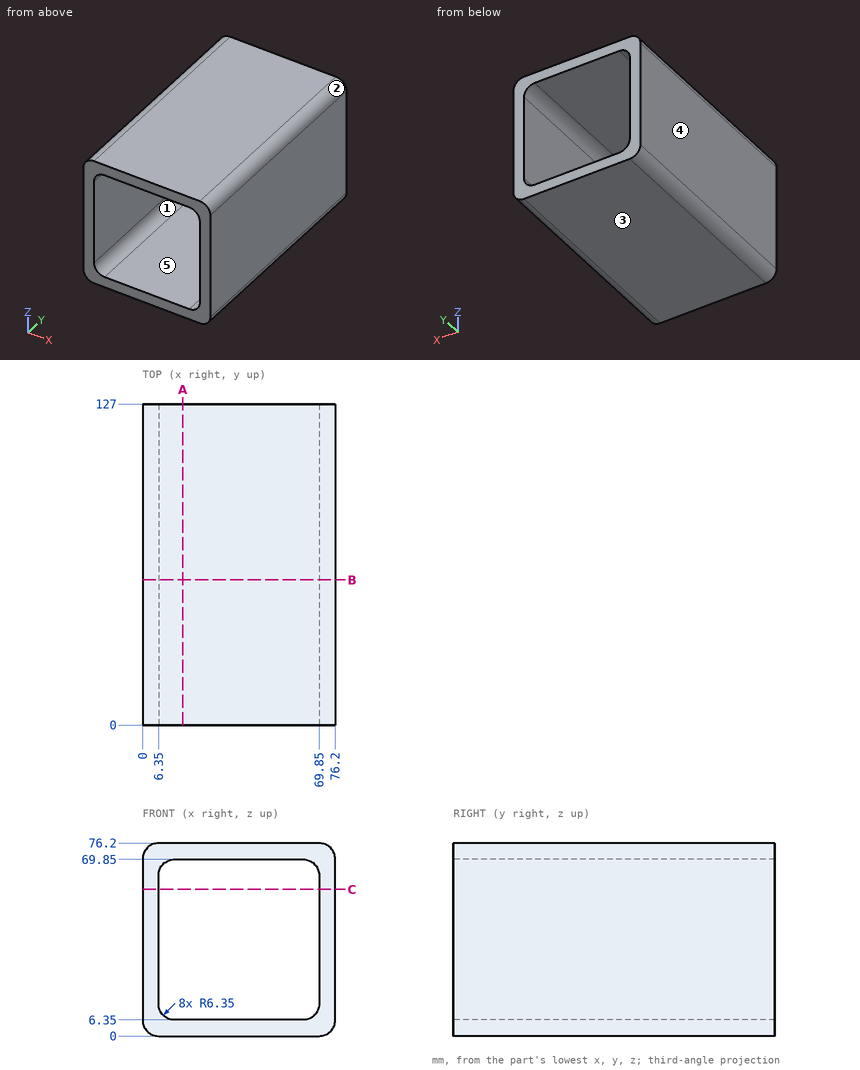
Study the drawing (mm; zero at the part's minimum x, y, z) and answer. A direction names the side the tool comes from. Round coordinates to 2 decimals unless told otherwise and drop trailing zeros. Write each loop counter-clockwise with the first axis right and the second up, starting at its lowest first coordinate (ties: lowest second). Pieces come first, ordered by that corner, then holes.
1) The mould has two halves that part along Z. Classify the marked faces 1, 2 and 3: pulls with the +Z half, pulls with the -Z half, needs draft (parallel to the pull), parting line crosses it, or undercut.
2) A cutting plane is placed at A-A (x = 16). Give the vertices of the cut face in (y, z).
3) Straight lines are drawn through the part: line 1 (Z direction, x = 29.5, y = 109); line 2 (Z direction, x = 11, y = 98.5). For each, find the intervals that lie inside material, in ascending order.
4) A cutting plane is placed at C-C (z = 58). Give the vertices of the cut face in (x, y).
5) A cutting plane is placed at B-B (y = 57.5). Give the vertices of the cut face in (x, z).
6) A tool of negligible diameter and unlimited length cuts with its end or side. For the marked faces 4 and 5, from which of +Z, -Z, +X, -X, +Y, -Y can it reach the whole face along a straight path? Write none if from no direction.
Completed:
1. face 1: undercut
1. face 2: pulls with the +Z half
1. face 3: pulls with the -Z half
2. outline: (0, 0) - (127, 0) - (127, 6.35) - (0, 6.35) - close; (0, 69.85) - (127, 69.85) - (127, 76.2) - (0, 76.2) - close
3. line 1: z = 0 to 6.35, 69.85 to 76.2
3. line 2: z = 0 to 6.58, 69.62 to 76.2
4. outline: (0, 0) - (6.35, 0) - (6.35, 127) - (0, 127) - close; (69.85, 0) - (76.2, 0) - (76.2, 127) - (69.85, 127) - close
5. outline: (0, 6.35) arc R6.35 ccw to (6.35, 0) - (69.85, 0) arc R6.35 ccw to (76.2, 6.35) - (76.2, 69.85) arc R6.35 ccw to (69.85, 76.2) - (6.35, 76.2) arc R6.35 ccw to (0, 69.85) - close; hole (6.35, 12.7) arc R6.35 ccw to (12.7, 6.35) - (63.5, 6.35) arc R6.35 ccw to (69.85, 12.7) - (69.85, 63.5) arc R6.35 ccw to (63.5, 69.85) - (12.7, 69.85) arc R6.35 ccw to (6.35, 63.5) - close
6. face 4: +Z, -Z, -X, +Y, -Y
6. face 5: +Y, -Y
